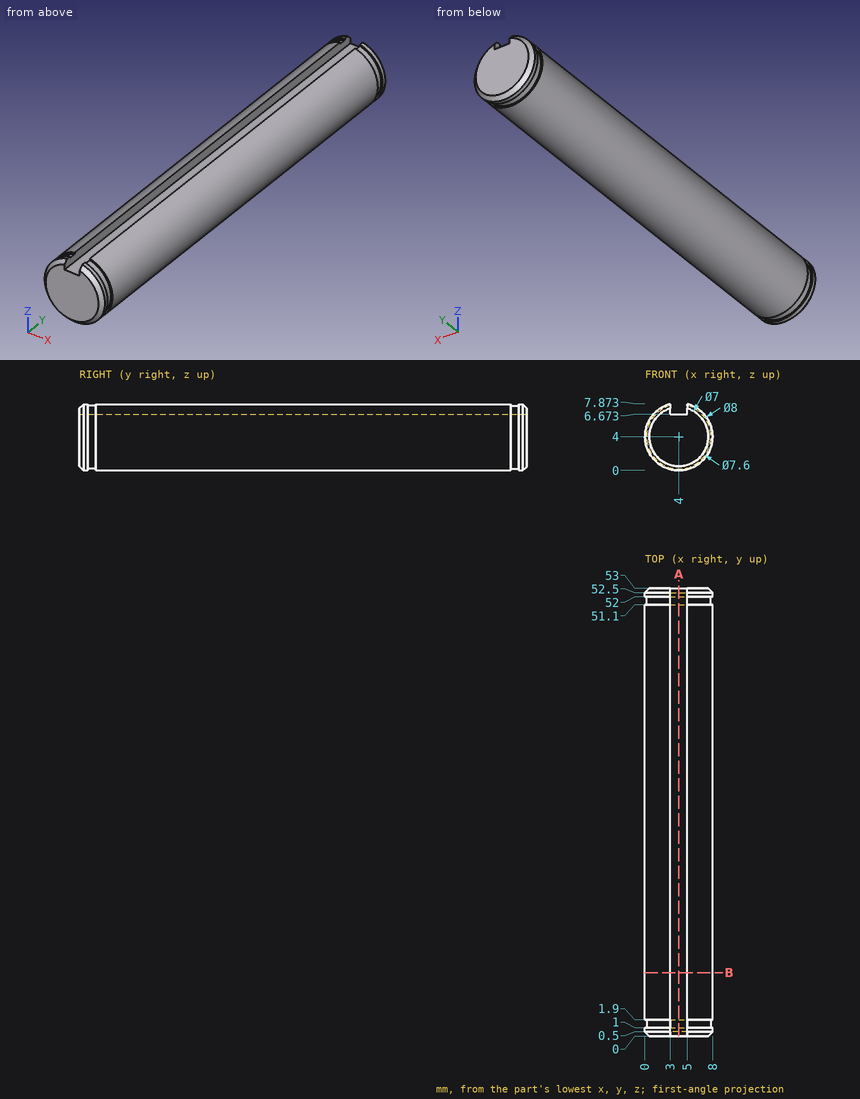
Answer from the drawing. Dimensions are ordinates in mm from the lowest x, y and z of the part. Round coordinates to 2 decimals unless told otherwise and drop trailing zeros. Loops run counter-clockwise (first coordinate to the right, second up) from the corner with the lowest first, then second, coordinate; pieces in that order, holes last.
Q1. Section A-A on x = 4 is taken. Write down the section's boundary in (y, z).
Q2. Consider probe 1 along Z at (x, y) = (4.25, 23.5); probe 2 along Z at (x, y) = (5.25, 27.5); probe 3 along X at (y, z) = (47, 5). Determine where each line is inside the solid, lowest interval first.
Q3. Each of these flat-tipped pins is pushed along its axis until it touches: pin 1 (2 mm diameter, centred on x = 3.5, y = 18, fed in from +Z); pin 2 (4 mm diameter, centred on y = 33.5, z = 7, fed in from +X); pin 3 (1 mm diameter, centred on y = 20, z = 7.5, fed in from -X). Where does it stop, or does it pass through?
Q4. Section B-B on y = 7.5 is taken. Write down the section's boundary in (x, z), and give its area (3 significant figures).
Output:
1. outline: (0, 0.5) - (0.5, 0) - (1, 0) - (1, 0.2) - (1.9, 0.2) - (1.9, 0) - (51.1, 0) - (51.1, 0.2) - (52, 0.2) - (52, 0) - (52.5, 0) - (53, 0.5) - (53, 6.67) - (0, 6.67) - close
2. probe 1: z = 0.01 to 6.67
2. probe 2: z = 0.2 to 7.8
2. probe 3: x = 0.13 to 7.87
3. pin 1: stops at z = 7.87
3. pin 2: stops at x = 7.87
3. pin 3: stops at x = 1.35
4. outline: (3, 6.67) - (3, 7.87) arc R4 ccw (long way) to (5, 7.87) - (5, 6.67) - close
4. area: 47.7 mm2
